Autodesk Inventor part; units mm, degrees
ref_plane "YZ Plane" through (0, 0, 0) normal (1, 0, 0) x (0, 1, 0)
ref_plane "XZ Plane" through (0, 0, 0) normal (0, 1, 0) x (-1, 0, 0)
ref_plane "XY Plane" through (0, 0, 0) normal (0, 0, 1) x (1, 0, 0)
sketch "Base Profile" plane through (0, 0, 0) normal (0, 1, 0) x (-1, 0, 0)
  line L0 (0, 0) -> (15, 0)
  line L1 (15, 0) -> (15, -15)
  line L2 (15, -15) -> (0, -15)
  line L3 (0, -15) -> (0, 0)
  line L4 (15, 0) -> (32, 0)
  line L5 (32, 0) -> (32, -15)
  line L6 (32, -15) -> (15, -15)
  line L7 (15, -15) -> (15, 0)
  dimension "d164" = 15
  dimension "d165" = 15
  dimension "d166" = 17
  dimension "d167" = 15
extrude "Stock" add sketch "Base Profile" against normal blind 33
extrude "Extrusion Post" add sketch "Base Profile" along normal blind 15 contours L0 L1 L2 L3
sketch "Side Profile" plane through (0, -33, -15) normal (0, 0, -1) x (-1, 0, 0)
  line L0 (0, 0) -> (0, 48)
  line L1 (32, 0) -> (0, 0)
  line L2 (32, 33) -> (32, 0)
  line L3 (15, 33) -> (32, 33)
  line L4 (15, 33) -> (15, 48)
  line L5 (0, 48) -> (15, 48)
  line L6 (0, 16.5) -> (32, 16.5)
  line L7 (0, 25.5) -> (32, 25.5)
  line L8 (15, 33) -> (15, 0)
  point P0 (15, 16.5)
  point P1 (15, 25.5)
  dimension "d354" = 7.5
  dimension "d355" = 16.5
extrude "Lower Half Cut" cut sketch "Side Profile" against normal through all contours L8 L7 L2 L6
sketch "Bottom Profile" plane through (-35, 0, -15) normal (0, -1, 0) x (1, 0, 0)
  line L0 (13.5, 7.5) -> (9.5, 7.5) construction
  line L1 (13.5, 10.675) -> (9.5, 10.675)
  line L2 (9.5, 4.325) -> (13.5, 4.325)
  arc A0 (13.5, 4.325) -> (13.5, 10.675) centre (13.5, 7.5) ccw
  arc A1 (9.5, 10.675) -> (9.5, 4.325) centre (9.5, 7.5) ccw
  line L3 (3, 15) -> (3, 0)
  line L4 (35, 15) -> (3, 15)
  point P0 (11.5, 7.5)
  dimension "d291" = 4
  dimension "d292" = 6.35
  dimension "d293" = 6.5
  dimension "d294" = 7.5
extrude "Slot Cut" cut sketch "Bottom Profile" along normal blind 24
sketch "Front Hole Pattern" plane through (0, -33, 0) normal (1, 0, 0) x (0, 0, -1)
  line L0 (0, 0) -> (0, 48)
  circle A0 centre (7.5, 40.5) radius 3.175
  line L1 (0, 48) -> (15, 48)
  circle A1 centre (7.5, 30.25) radius 3.175
  dimension "d317" = 6.35
  dimension "d318" = 7.5
  dimension "d319" = 7.5
  dimension "d368" = 17.75
hole "Front Mounting Hole" at (0, 7.5, -7.5) direction (-1, 0, 0) diameter 3.2004 end through all counterbore diameter 6.35 counterbore depth 10.675
sketch "Sketch33" plane through (0, 15, 0) normal (0, 1, 0) x (1, 0, 0)
  line L0 (-15, 15) -> (-15, 0)
  line L1 (-15, 0) -> (0, 0)
  line L2 (0, 0) -> (0, 15)
  line L3 (0, 15) -> (-15, 15)
  circle A0 centre (-7.5, 7.5) radius 3.175
  dimension "d340" = 6.35
  dimension "d341" = 7.5
  dimension "d342" = 7.5
hole "Top Mounting Hole" at (-7.5, 15, -7.5) direction (0, -1, 0) diameter 3.2004 end through all counterbore diameter 6.35 counterbore depth 25.5044
hole "Front Adjustment Hole" at (0, -2.75, -7.5) direction (-1, 0, 0) diameter 3.2004 end through all counterbore diameter 6.35 counterbore depth 10.675
sketch "Rear Hole Patttern" plane through (-32, -33, -15) normal (-1, 0, 0) x (0, 0, 1)
  line L0 (0, 25.5) -> (15, 25.5) construction
  line L1 (15, 33) -> (15, 25.5) construction
  line L2 (0, 33) -> (15, 33) construction
  line L3 (0, 33) -> (0, 25.5) construction
  line L4 (15, 16.5) -> (0, 16.5) construction
  line L5 (0, 16.5) -> (0, 0) construction
  line L6 (15, 0) -> (0, 0) construction
  line L7 (15, 16.5) -> (15, 0) construction
  circle A0 centre (7.5, 30.25) radius 1.5
  circle A1 centre (7.5, 11.75) radius 1.5
  line L8 (0, 27.5) -> (15, 27.5) construction
  line L9 (0, 16.5) -> (0, 0)
  line L10 (0, 14.5) -> (15, 14.5) construction
  dimension "d357" = 3
  dimension "d358" = 7.5
  dimension "d360" = 3
  dimension "d362" = 7.5
  dimension "d364" = 2
  dimension "d365" = 2
  dimension "d366" = 2.75
  dimension "d367" = 2.75
hole "Rear Holes" at (-32, -21.25, -7.5) direction (1, 0, 0) diameter 2.459 depth 13.6652 tip angle 118
fillet "Fillet" radius 6.35 2 edges at (-32, -3.75, -15) (-32, -24.75, -15)
equation "\"d164\" = extrusionWidth"
equation "\"d165\" = extrusionWidth"
equation "\"d166\" = idlerLength"
equation "\"d167\" = d165"
equation "\"d168\" = extrusionOffset"
equation "\"extrusionWidth\" = 15"
equation "\"idlerLength\" = 17"
equation "\"bearingOffsetFromBottom\" = 7.5"
equation "\"extrusionOffset\" = 33"
equation "\"bearingStackHeight\" = 9"
equation "\"bearingSlotLength\" = 4"
equation "\"bearingClearance\" = 13"
equation "\"pinSupportLength\" = 2"
properties part number "B Idler (Tulip)" material "Aluminum 6061"
Geometry check sheet. Reference: the model listing, model coordinates, mm. A direction names the side the tool comes from. Round coordinates to 2 decimals unless told otherwise and drop trailing zeros. Order: outer loops, then holes, each group sorted by start corner. A loop starts at its lowest first (then second) coordinate and runs counter-clockwise, first axis right, second up. Notation, with made-up numbers: M 71.25,74 L 117.25,74 A12 cw 117.25,81 Z; hole C 76,37 d10. An arc over 180 degrees is marked long. Answer as CSV lines item,"result".
1) Gauge pin test, flat ends, axial feed: pin 1 Ø3.5 at (x, z) = (-7.5, -7.5) entering from +Y; pin 2 Ø5 at (y, z) = (7.5, -7.5) entering from -X; pin 3 Ø4 at (y, z) = (-1.5, -13) entering from -X; pin 4 Ø6 at (x, y) = (-19, 9) entering from +Z. Record the tip position at first contact, or that the pin passes through.
Entries:
pin 1,"y = -10.5"
pin 2,"x = -15"
pin 3,"x = -31.55"
pin 4,"through"
2) Mould release check, pull along Y, two halves, no side actions. Record for faces 5 (the face through (0, -9, -8)), 6 (the face through (-16, -33, -7)), 7 (the face through (-12.87, 6.42, -6.32)), 8 (the face through (-9.8, -2.773, -4.325)): +Y half, -Y half, draft (parallel to the pull), parting line (faces both ways), or undercut.
Entries:
face 5,"draft"
face 6,"-Y half"
face 7,"undercut"
face 8,"undercut"
3) Sectioned sample at D-D on y = -8. Record the cut outline in (x, z) (3 decimals).
Entries:
outline,"M -15,-15 L 0,-15 L 0,0 L -15,0 Z; hole C -7.5,-7.5 d6.35"
4) Sectioned sample at C-C on y = 8. Record the cut outline in (x, z) (3 decimals), and give its area (3 significant figures).
Entries:
outline,"M -15,-15 L 0,-15 L 0,-10.635 L -7,-10.635 A3.175 cw -8,-10.635 L -10.675,-10.635 L -10.675,-9.02 L -15,-9.02 Z; M -15,-5.98 L -10.675,-5.98 L -10.675,-4.365 L -8,-4.365 A3.175 cw -7,-4.365 L 0,-4.365 L 0,0 L -15,0 Z"
area,"145 mm2"
5) Thickness scan on probe 1 along Y at (x, z) = (-11.6, -7.5); probe 2 along Y at (x, z) = (-2.25, -7.5) (3 decimals); probe 3 along Z at (x, y) = (-7.5, 9.5) (3 decimals). Record the ranges inside material, lowest first. Write a range as [from, to].
Entries:
probe 1,"[-33, -4.35], [-1.15, 5.9], [9.1, 15]"
probe 2,"[-33, -5.925], [0.425, 4.325], [10.675, 15]"
probe 3,"[-15, -10.675], [-4.325, 0]"
6) Sectioned sample at B-B on z = -1.75. Record the cut outline in (x, y).
Entries:
outline,"M -32,-33 L 0,-33 L 0,15 L -15,15 L -15,0 L -32,0 L -32,-7.5 L -15,-7.5 L -15,-16.5 L -32,-16.5 Z"
7) Tool access check on faces 1 (the face through (-24, -20, -10.675)), 2 (the face through (-2.97, 9.43, -4.98)), 3 (the face through (-30.19, -21.3, -8.73)), 4 (the face through (-32, -4, -4)). Record the directions out of +Z, -Z, +X, -X, +Y, -Y that give a thin tool (end or side, any length) a straight path to the whole face; none if there is none.
Entries:
face 1,"+Y"
face 2,"+X"
face 3,"-X"
face 4,"+Z, -Z, -X, +Y, -Y"
8) Sectioned sample at A-A on y = -19. Record the cut outline in (x, z) (3 decimals), and give its area (3 significant figures).
Entries:
outline,"M -32,-8.65 A6.35 ccw -25.65,-15 L 0,-15 L 0,0 L -32,0 Z; hole M -25.5,-10.675 L -21.5,-10.675 A3.175 ccw -21.5,-4.325 L -25.5,-4.325 A3.175 ccw Z; hole C -7.5,-7.5 d3.2"
area,"406 mm2"
